Can you work these out from the model? Positions are in its coordinate system, mm. Face numbers are marked on the shaded views. A direction names the side the tool comes from. Give positions to 0.01 mm unless a question says otherwise; leave off trailing zeros. Loops run counter-clockwise (first coordinate to the right, second up) from the corner with the lowest first, then second, coordinate; pieces in that order, holes last. Notation, with made-up numbers: (5, 55.25) - (13, 55.25) arc R19 cw to (13, 59.25) - close; hole circle Ø2 at (46, 85). An arc over 180 degrees is marked (long way). Write item = value, one per line.
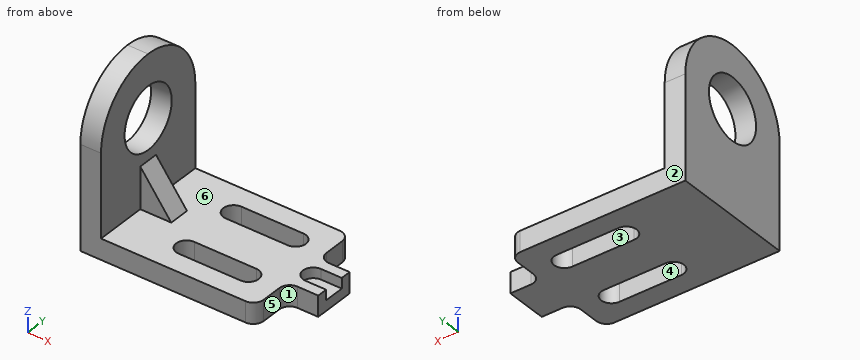
from build123d import *

# Parameters (mm, degrees)
F1_DEPTH = 203.2
F2_DEPTH = 25.4
F3_DEPTH = 12.7
F0_W     = 38.1
F0_H     = 25.4
F4_DEPTH = 76.2
F6_R     = 76.19999
F7_D     = 76.2
F8_SIZE2 = 38.09999
F8_SIZE  = 50.79999


# Not quite as in the source:
# - a fillet or chamfer is up to 0.001 mm smaller than in the source, because OpenCascade refuses the exact size


with BuildPart() as f1:
    # F0 (on Top) → F1 (new body)
    with BuildSketch(Plane.XY):
        Polygon((25.4, 0), (0, 0), (0, -152.4), (25.4, -152.4), (25.4, -88.9), (25.4, -63.5), align=None)
    extrude(amount=F1_DEPTH)

    # F0 (on Top) → F2 (join)
    with BuildSketch(Plane.XY):
        with BuildLine():
            Line((101.6, 0), (25.4, 0))
            Line((25.4, 0), (25.4, -63.5))
            Line((25.4, -63.5), (63.5, -63.5))
            Line((63.5, -63.5), (63.5, -88.9))
            Line((63.5, -88.9), (25.4, -88.9))
            Line((25.4, -88.9), (25.4, -152.4))
            Line((25.4, -152.4), (101.6, -152.4))
            Line((101.6, -152.4), (203.2, -152.4))
            ThreePointArc((203.2, -152.4), (212.1802561211, -148.6802561211), (215.9, -139.7))
            Line((215.9, -139.7), (215.9, -114.3))
            ThreePointArc((215.9, -114.3), (219.6197438789, -105.3197438789), (228.6, -101.6))
            Line((228.6, -101.6), (254, -101.6))
            Line((254, -101.6), (254, -88.9))
            Line((254, -88.9), (228.6, -88.9))
            ThreePointArc((228.6, -88.9), (215.9, -76.2), (228.6, -63.5))
            Line((228.6, -63.5), (254, -63.5))
            Line((254, -63.5), (254, -50.8))
            Line((254, -50.8), (228.6, -50.8))
            ThreePointArc((228.6, -50.8), (219.6197438789, -47.0802561211), (215.9, -38.1))
            Line((215.9, -38.1), (215.9, -12.7))
            ThreePointArc((215.9, -12.7), (212.1802561211, -3.7197438789), (203.2, 0))
            Line((203.2, 0), (101.6, 0))
        make_face()
        with BuildLine():
            Line((177.8, -127), (101.6, -127))
            ThreePointArc((101.6, -127), (88.9, -114.3), (101.6, -101.6))
            Line((101.6, -101.6), (177.8, -101.6))
            ThreePointArc((177.8, -101.6), (190.5, -114.3), (177.8, -127))
        make_face(mode=Mode.SUBTRACT)
        with BuildLine():
            ThreePointArc((101.6, -50.8), (88.9, -38.1), (101.6, -25.4))
            Line((101.6, -25.4), (177.8, -25.4))
            ThreePointArc((177.8, -25.4), (190.5, -38.1), (177.8, -50.8))
            Line((177.8, -50.8), (101.6, -50.8))
        make_face(mode=Mode.SUBTRACT)
    extrude(amount=F2_DEPTH)

    # F0 (on Top) → F3 (join)
    with BuildSketch(Plane.XY):
        Polygon((254, -88.9), (254, -63.5), (228.6, -63.5), (228.6, -76.2), (228.6, -88.9), align=None)
        with BuildLine():
            Line((228.6, -76.2), (228.6, -63.5))
            ThreePointArc((228.6, -63.5), (215.9, -76.2), (228.6, -88.9))
            Line((228.6, -88.9), (228.6, -76.2))
        make_face()
    extrude(amount=F3_DEPTH)

    # F0 (on Top) → F4 (join)
    with BuildSketch(Plane.XY):
        with Locations((44.45, -76.2)):
            Rectangle(F0_W, F0_H)
    extrude(amount=F4_DEPTH)

    # F6 (radius 76.2 in the source; OpenCascade refuses exactly that, so slightly less here)
    f6_edges = [f1.edges().sort_by_distance(p)[0] for p in [
        (12.7, -152.4, 203.2),
        (12.7, 0, 203.2),
    ]]
    fillet(f6_edges, radius=F6_R)

    # F7 (through all)
    with Locations(Plane(origin=(0, 0, 0), x_dir=(0, 1, 0), z_dir=(-1, 0, 0))):
        with Locations((-76.2, -127)):
            Hole(F7_D / 2)

    # F8 (size 50.8 and 38.0999999365 in the source; OpenCascade refuses exactly that, so slightly less here)
    f8_edges = [f1.edges().sort_by_distance(p)[0] for p in [
        (63.5, -76.2, 76.2),
    ]]
    f8_side = f1.faces().sort_by_distance((63.5, -76.2, 50.8))[0]
    chamfer(f8_edges, length=F8_SIZE, length2=F8_SIZE2, reference=f8_side)


solid = f1.part
Q1. I need wall thicknesses on L1, parallel to Y at x = 44.5, z = 28.5; L2, parallel to X at y = -32.5, z = 36.5. Which ranges of each line are inside material? Lowest first, please.
Output:
L1 = -88.9 to -63.5
L2 = 0 to 25.4
Q2. Imagine slicing it at A-A, the plane x = 126. Write out the boundary of the cut face in (y, z), then the cut area to 3 significant figures.
Output:
outline = (-152.4, 0) - (-127, 0) - (-127, 25.4) - (-152.4, 25.4) - close; (-101.6, 0) - (-50.8, 0) - (-50.8, 25.4) - (-101.6, 25.4) - close; (-25.4, 0) - (0, 0) - (0, 25.4) - (-25.4, 25.4) - close
area = 2,580 mm2
Q3. Imagine slicing it at B-B, the plane z = 55. Write out the boundary of the cut face in (x, y).
Output:
outline = (0, -152.4) - (25.4, -152.4) - (25.4, -88.9) - (41.3, -88.9) - (41.3, -63.5) - (25.4, -63.5) - (25.4, 0) - (0, 0) - close
Q4. Imagine slicing it at D-D, the plane z = 148. Write out the boundary of the cut face in (x, y), then the cut area to 3 significant figures.
Output:
outline = (0, -149.45) - (25.4, -149.45) - (25.4, -107.99) - (0, -107.99) - close; (0, -44.41) - (25.4, -44.41) - (25.4, -2.95) - (0, -2.95) - close
area = 2,110 mm2
Q5. We'd pull the mould along Y, two halves only. Please class the marked faces 1, 2 and 3: released by +Y, released by -Y, zero draft, split by the parting line, or undercut.
Output:
face_1 = released by -Y
face_2 = released by +Y
face_3 = undercut
Q6. Which directions (+Z, -Z, +X, -X, +Y, -Y) give clear straight access to the entire face, cutting with the end or side of a thin tool? Please do the marked faces 4, 5 and 6.
Output:
face_4 = +Z, -Z
face_5 = +Z, -Z, +X, -Y
face_6 = +Z, +X
Q7. For pin 1 (12.5 mm diameter, centred on y = -31, z = 8.5, fed in from +X); pin 2 (10 mm diameter, centred on y = -96.5, z = 73.5, fed in from +X); pin 3 (6.5 mm diameter, centred on x = 245, z = 22, fed in from +Y), each with a flat end and sliding along its axis, tell me the tip position at first contact or that it passes through.
Output:
pin_1 = 215.9
pin_2 = 25.4
pin_3 = -50.8
